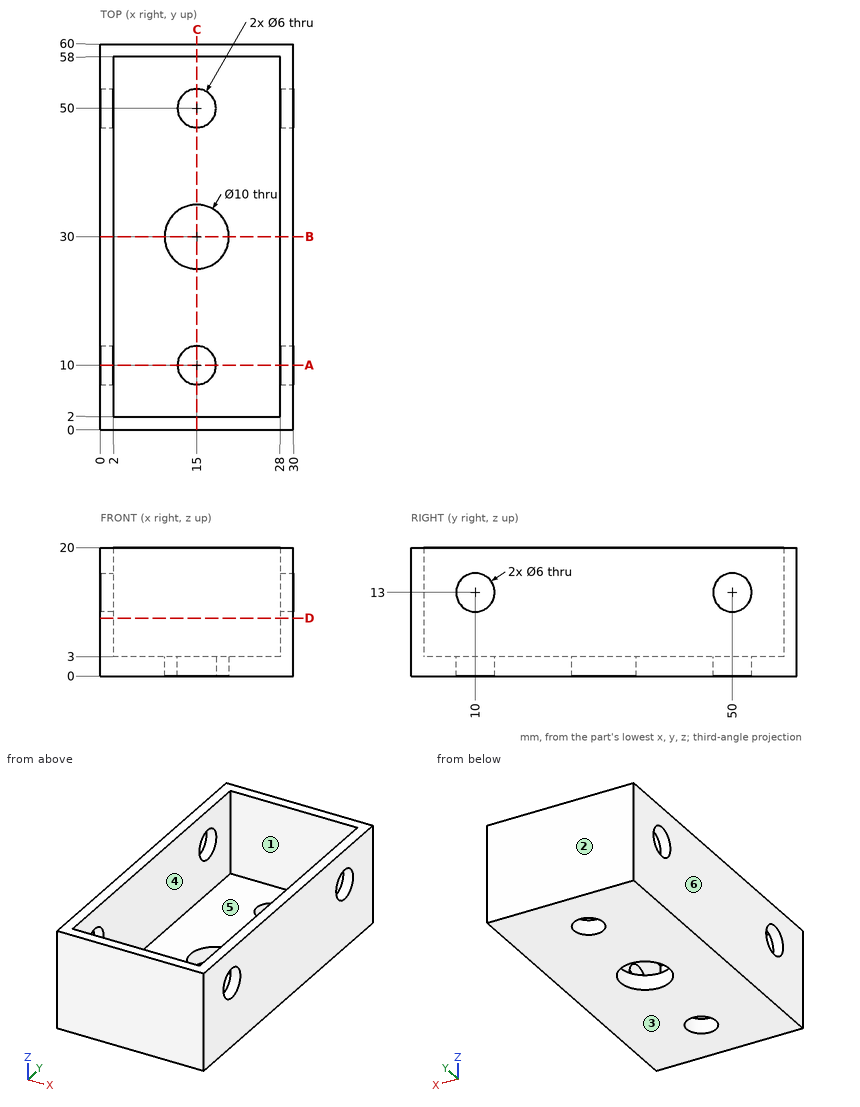
Study the drawing (mm; zero at the part's minimum x, y, z) and answer. A direction names the side the tool comes from. Coordinates: 2 decimals unless noted, no trailing zeros. Write each loop counter-clockwise with the first axis right and the second up, starting at its lowest first coordinate (ties: lowest second). Pieces come first, ordered by that corner, then holes. Notation, with made-up numbers: (-19, 68.25) - (30, 68.25) arc R32 ccw to (30, 96.25) - close; hole circle Ø5 at (-29.5, 53). An arc over 180 degrees is marked (long way). Answer as a JSON object with one key per item and string values.
Q1. Which of the six approach directions +Z, -Z, +X, -X, +Y, -Y give full straight-line access (tool end or side, diameter ignored) to the marked faces 5 and 6?
Results list:
{"face 5": "+Z", "face 6": "+Z, -Z, -X, +Y, -Y"}
Q2. Given pin 1 Ø5 at (x, y) = (14, 41) entering from +Z; pin 2 Ø5 at (x, y) = (15, 10) entering from +Z, each flat-ended and moving along its own axis, determine where each tip first touches the part or whether it passes through.
Results list:
{"pin 1": "stops at z = 3", "pin 2": "passes through"}
Q3. Find section A-A (y = 10). Write down the section's boundary in (x, z).
Results list:
{"outline": "(0, 0) - (12, 0) - (12, 3) - (2, 3) - (2, 10) - (0, 10) - close; (0, 16) - (2, 16) - (2, 20) - (0, 20) - close; (18, 0) - (30, 0) - (30, 10) - (28, 10) - (28, 3) - (18, 3) - close; (28, 16) - (30, 16) - (30, 20) - (28, 20) - close"}
Q4. Consider L1, parallel to Y at x = 1.6, z = 13; L2, parallel to Y at x = 15, z = 2.1; L3, parallel to X at y = 26, z = 4.5. Determine where each line is inside the solid, lowest interval first. Write a range as from..to.
Results list:
{"L1": "y = 0..7, 13..47, 53..60", "L2": "y = 0..7, 13..25, 35..47, 53..60", "L3": "x = 0..2, 28..30"}
Q5. Find section B-B (y = 30). Write down the section's boundary in (x, z).
Results list:
{"outline": "(0, 0) - (10, 0) - (10, 3) - (2, 3) - (2, 20) - (0, 20) - close; (20, 0) - (30, 0) - (30, 20) - (28, 20) - (28, 3) - (20, 3) - close"}
Q6. For a pull along Y with two mould halves and no side action, classify the marked faces 1, 2, 3 and 4 as pulls with the +Y half, pulls with the -Y half, needs draft (parallel to the pull), parting line crosses it, or undercut.
Results list:
{"face 1": "undercut", "face 2": "pulls with the +Y half", "face 3": "needs draft", "face 4": "undercut"}
Q7. Find section D-D (z = 9). Write down the section's boundary in (x, y).
Results list:
{"outline": "(0, 0) - (30, 0) - (30, 60) - (0, 60) - close; hole (2, 2) - (28, 2) - (28, 58) - (2, 58) - close"}
Q8. Find section C-C (x = 15). Write down the section's boundary in (y, z), plus the area to 3 significant figures.
Results list:
{"outline": "(0, 0) - (7, 0) - (7, 3) - (2, 3) - (2, 20) - (0, 20) - close; (13, 0) - (25, 0) - (25, 3) - (13, 3) - close; (35, 0) - (47, 0) - (47, 3) - (35, 3) - close; (53, 0) - (60, 0) - (60, 20) - (58, 20) - (58, 3) - (53, 3) - close", "area": "182 mm^2"}
